Work out the finished part from the listing and answer in its coordinate system (mm). Face numbers are marked on the shaded views. A direction names the side the tool comes from. Give positions to 0.01 mm unless a question says otherwise; leave off trailing zeros. Order: outer loops, then holes, each group sorted by start corner. A loop starts at its lowest first (then second) coordinate and runs counter-clockwise, first axis right, second up. Notation, with made-up numbers: (10, 38) -> (51, 38) arc R21 ccw to (51, 72) -> close; hole circle Ø6 at (44, -3). An arc over 180 degrees is marked (long way). Answer as CSV lines item,"result". Start each with the question number.
1. A cutting plane is placed at B-B (y = 20). Give the vertices of the cut face in (x, z), then the cut area to 3 significant figures.
2. A cutting plane is placed at A-A (y = 29.5). Give the vertices of the cut face in (x, z).
3. For a pull along Z with two mould halves and no side action, classify the marked faces 1, 2 and 3 as released by +Z, released by -Z, zero draft, split by the parting line, or undercut.
4. Find the intervals of material crossed by L1, parallel to X at y = 1.1, z = 0; L2, parallel to X at y = 2, z = 0; L3, parallel to Y at x = 5.5, z = -8.5, in increasing order.
5. Flat-ended cylindrical pins translate along their axes: pin 1 (2.5 mm diameter, centred on x = 6.3, z = 0, fed in from +Y); pin 2 (1 mm diameter, centred on x = 6, z = -0.5, fed in from -Y); pin 3 (1.5 mm diameter, centred on y = 9.5, z = -6, fed in from +X); pin 4 (6.5 mm diameter, centred on x = 0, z = 0, fed in from +Y). Find the tip coordinate at first contact, or state that the pin passes through.
6. For the marked faces 4 and 5, determine the directions among +Z, -Z, +X, -X, +Y, -Y from which every point of the face is accessible in a straight line to the end or side of a thin tool.
from build123d import *

# Parameters (mm, degrees)
CHAMFER_1_SIZE           = 1
SKETCH_2_R               = 1.6
CUT_EXTRUDE_1_DEPTH      = 3.2
EXTRUDE_START            = 5.5
SKETCH_3_R               = 10.2
SKETCH_3_R_2             = 8.35
EXTRUDE_1_DEPTH          = 5.5
CHAMFER_2_SIZE           = 0.5
CUT_EXTRUDE_2_DEPTH      = 39.417183655
CUT_EXTRUDE_2_DEPTH_BACK = 39.417183655
SKETCH_4_R               = 1.15


with BuildPart() as part:
    # 스케치1 → 회전1 (revolve)
    with BuildSketch(Plane(origin=(0, 0, 0), x_dir=(0, 0, -1), z_dir=(1, 0, 0))):
        Polygon((4.1, 0), (4.1, 35), (6, 35), (6, 25), (11.2, 10), (11.2, 8), (10.2, 8), (10.2, 5.7), (10.2, 4), (10.2, 0), align=None)
    revolve(axis=Axis((0, 0, 0), (0, 1, 0)))

    # 모따기1
    chamfer_1_edges = [part.edges().sort_by_distance(p)[0] for p in [
        (0, 35, 6),
    ]]
    chamfer(chamfer_1_edges, length=CHAMFER_1_SIZE)

    # 스케치2 → 컷-돌출1 (cut)
    with BuildSketch(Plane(origin=(0, 0, 0), x_dir=(1, 0, 0), z_dir=(0, 1, 0))):
        with Locations(Location((-6.3, 0, 0), (0, 0, 270))):
            Circle(SKETCH_2_R)
        with Locations(Location((6.3, 0, 0), (0, 0, 90))):
            Circle(SKETCH_2_R)
    extrude(amount=CUT_EXTRUDE_1_DEPTH, mode=Mode.SUBTRACT)

    # 스케치3 → 보스-돌출1 (add)
    with BuildSketch(Plane.XZ.offset(EXTRUDE_START)):
        with Locations(Location((0, 0, 0), (0, 0, 270))):
            Circle(SKETCH_3_R)
        with Locations(Location((0, 0, 0), (0, 0, 270))):
            Circle(SKETCH_3_R_2, mode=Mode.SUBTRACT)
    extrude(amount=-EXTRUDE_1_DEPTH)

    # 모따기2
    chamfer_2_edges = [part.edges().sort_by_distance(p)[0] for p in [
        (0, 0, 4.1),
    ]]
    chamfer(chamfer_2_edges, length=CHAMFER_2_SIZE)

    # 스케치4 → 컷-돌출2 (cut, two sides: drawn at the far end of the back side and taken through both)
    with BuildSketch(Plane(origin=(0, 0, 0), x_dir=(0, 0, -1), z_dir=(1, 0, 0)).offset(-CUT_EXTRUDE_2_DEPTH_BACK)):
        with Locations((0, -5.5)):
            Circle(SKETCH_4_R)
    extrude(amount=CUT_EXTRUDE_2_DEPTH + CUT_EXTRUDE_2_DEPTH_BACK, mode=Mode.SUBTRACT)

    # 스케치6 → 컷-회전1 (revolve, cut)
    with BuildSketch(Plane(origin=(0, 0, 0), x_dir=(0, 0, -1), z_dir=(1, 0, 0)), mode=Mode.PRIVATE) as cut_revolve_1_sk:
        Polygon((10.2, 5), (9.7, 4.5), (9.7, 4), (10.2, 3.5), (11.2, 3.5), (11.2, 5), align=None)
        Polygon((9.7, 1.5), (9.7, 1), (10.2, 0.5), (11.2, 0.5), (11.2, 2), (10.2, 2), align=None)
        Polygon((9.7, -1.5), (9.7, -2), (10.2, -2.5), (11.2, -2.5), (11.2, -1), (10.2, -1), align=None)
    revolve(cut_revolve_1_sk.sketch.rotate(Axis((0, 0, 0), (0, -1, 0)), 180), axis=Axis((0, 0, 0), (0, -1, 0)), mode=Mode.SUBTRACT)

    # 모따기3: read off the stored shape, not the designer's step
    # 모따기3 outline → 모따기3 (revolve, cut)
    with BuildSketch(Plane.XY):
        Polygon((10.2, -5.3), (10, -5.5), (10.2, -5.5), align=None)
    revolve(axis=Axis((0, 0, 0), (0, 1, 0)), mode=Mode.SUBTRACT)


solid = part.part
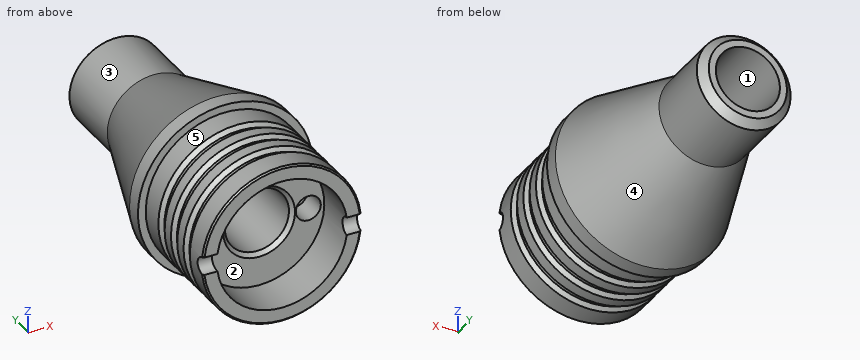
Answer sheet:
1,outline,"circle Ø15.47 at (0, 0); hole circle Ø8.2 at (0, 0)"
1,area,"135 mm^2"
2,outline,"circle Ø12 at (0, 0); hole circle Ø8.2 at (0, 0)"
3,face 1,"undercut"
3,face 2,"undercut"
3,face 3,"split by the parting line"
4,L1,"x = -9.7 to -7.9, -4.7 to -4.1, 4.1 to 4.7, 7.9 to 9.7"
4,L2,"x = -10.2 to -7.9, -4.7 to -4.1, 4.1 to 4.7, 7.9 to 10.2"
4,L3,"y = -5.38 to -2.42, -1.08 to 0.58, 1.92 to 3.58, 4.92 to 13.1"
5,pin 1,"stops at y = 34.95"
5,pin 2,"stops at y = 3.2"
5,pin 3,"stops at x = 9.89"
5,pin 4,"passes through"
6,face 4,"+Y"
6,face 5,"-Y"
